from build123d import *

# Parameters (mm, degrees)
F0_W      = 25.4
F0_H      = 50.8
F1_DEPTH  = 50.8
F2_W      = 35.56
F2_H      = 35.56
F3_DEPTH  = 12.7
F4_W      = 17.145
F4_H      = 8.255
F4_H_2    = 6.858
F5_DEPTH  = 7.62
F6_W      = 17.145
F6_H      = 8.255
F6_H_2    = 6.858
F7_DEPTH  = 7.62
F8_W      = 17.145
F8_H      = 35.56
F9_DEPTH  = 7.62
F10_W     = 17.145
F10_H     = 35.56
F11_DEPTH = 7.62


with BuildPart() as f1:
    # F0 (on Front) → F1 (new body)
    with BuildSketch(Plane.XZ):
        with Locations((12.7, 25.4)):
            Rectangle(F0_W, F0_H)
    extrude(amount=F1_DEPTH)

    # F2 (on face) → F3 (cut)
    with BuildSketch(Plane(origin=(0, 0, 0), x_dir=(0, -1, 0), z_dir=(-1, 0, 0))):
        with Locations((25.584483, 25.4)):
            Rectangle(F2_W, F2_H)
    extrude(amount=-F3_DEPTH, mode=Mode.SUBTRACT)

    # F4 (on face) → F5 (cut)
    with BuildSketch(Plane(origin=(0, 0, 0), x_dir=(-1, 0, 0), z_dir=(0, 1, 0))):
        with Locations((-8.5725, 46.6725)):
            Rectangle(F4_W, F4_H)
        with Locations((-8.5725, 32.258)):
            Rectangle(F4_W, F4_H_2)
        with Locations((-8.5725, 18.542)):
            Rectangle(F4_W, F4_H_2)
        with Locations((-8.5725, 4.1275)):
            Rectangle(F4_W, F4_H)
    extrude(amount=-F5_DEPTH, mode=Mode.SUBTRACT)

    # F6 (on face) → F7 (cut)
    with BuildSketch(Plane.XZ.offset(50.8)):
        with Locations((8.5725, 46.6725)):
            Rectangle(F6_W, F6_H)
        with Locations((8.5725, 32.258)):
            Rectangle(F6_W, F6_H_2)
        with Locations((8.5725, 18.542)):
            Rectangle(F6_W, F6_H_2)
        with Locations((8.5725, 4.1275)):
            Rectangle(F6_W, F6_H)
    extrude(amount=-F7_DEPTH, mode=Mode.SUBTRACT)

    # F8 (on face) → F9 (cut)
    with BuildSketch(Plane.XY.offset(50.8)):
        with Locations((8.5725, -25.4)):
            Rectangle(F8_W, F8_H)
    extrude(amount=-F9_DEPTH, mode=Mode.SUBTRACT)

    # F10 (on face) → F11 (cut)
    with BuildSketch(Plane(origin=(0, 0, 0), x_dir=(1, 0, 0), z_dir=(0, 0, -1))):
        with Locations((8.5725, 25.4)):
            Rectangle(F10_W, F10_H)
    extrude(amount=-F11_DEPTH, mode=Mode.SUBTRACT)


solid = f1.part
Build history of the part. All positions in model axes, mm. A direction names the side the tool comes from. Coordinates: 2 decimals unless noted, no trailing zeros. Order: outer loops, then holes, each group sorted by start corner. A loop starts at its lowest first (then second) coordinate and runs counter-clockwise, first axis right, second up. Notation, with made-up numbers: (79, -37) - (100, -37) arc R10 ccw to (100, -30) - close; hole circle Ø9 at (17, -7). An arc over 180 degrees is marked (long way). Write item = value, one per line. Start each with the question number.
1) Wall check: line 1 along Z through (x, y) = (8.75, -4) (3 decimals); line 2 along Y through (x, z) = (12, 26); line 3 along X through (y, z) = (-24.5, 40.5). Give the ranges that are in metal, low to high. Write a range as from..to.
2) Saw through at A-A on x = 5.25. Write the cut outline in (y, z) (3 decimals).
3) Flat gauge pins, fed straight in: pin 1 Ø4 at (y, z) = (-20.5, 8.5) entering from -X; pin 2 Ø2.5 at (x, y) = (6, -4) entering from +Z (3 decimals); pin 3 Ø2.5 at (y, z) = (-17, 48.5) entering from -X (3 decimals). Where does each tip first touch, or does it go through?
4) Saw through at B-B on y = -46. Write the cut outline in (x, z) (3 decimals), then the cut area to 3 significant figures.
5) Saw through at C-C on z = 27. Write the cut outline in (x, y).
6) Two-plate mould, pull along Y, no slides. Class faces 6 (the face through (12.7, -25, 26)), 7 (the face through (15, -43.18, 32)), 8 (the face through (17.145, -47, 32)): pulls with the +Y half, pulls with the -Y half, needs draft (parallel to the pull), parting line crosses it, or undercut.
7) Saw through at D-D on x = 14. Write the cut outline in (y, z) (3 decimals).
8) 3-axis set-ups, long thin cutter, end or side, ignore diameter. For faces 1 (the face through (8, -47, 28.829)), 2 (the face through (6, -43.364, 12)), 3 (the face through (9, -4, 28.829)), 4 (the face through (8, -47, 8.255)), 5 (the face through (14, -25, 7.62)): which of +Z, -Z, +X, -X, +Y, -Y reach the whole face in a straight line?
From the geometry:
q1.line_1 = 8.255..15.113, 21.971..28.829, 35.687..42.545
q1.line_2 = -50.8..-43.36, -7.8..0
q1.line_3 = 12.7..25.4
q2.outline = (-50.8, 8.255) - (-43.364, 8.255) - (-43.364, 15.113) - (-50.8, 15.113) - close; (-50.8, 21.971) - (-43.364, 21.971) - (-43.364, 28.829) - (-50.8, 28.829) - close; (-50.8, 35.687) - (-43.364, 35.687) - (-43.364, 42.545) - (-50.8, 42.545) - close; (-7.804, 7.62) - (-7.62, 7.62) - (-7.62, 8.255) - (0, 8.255) - (0, 15.113) - (-7.62, 15.113) - (-7.62, 21.971) - (0, 21.971) - (0, 28.829) - (-7.62, 28.829) - (-7.62, 35.687) - (0, 35.687) - (0, 42.545) - (-7.62, 42.545) - (-7.62, 43.18) - (-7.804, 43.18) - close
q3.pin_1 = 12.7
q3.pin_2 = 42.545
q3.pin_3 = 17.145
q4.outline = (0, 8.255) - (17.145, 8.255) - (17.145, 0) - (25.4, 0) - (25.4, 50.8) - (17.145, 50.8) - (17.145, 42.545) - (0, 42.545) - (0, 35.687) - (17.145, 35.687) - (17.145, 28.829) - (0, 28.829) - (0, 21.971) - (17.145, 21.971) - (17.145, 15.113) - (0, 15.113) - close
q4.area = 772 mm^2
q5.outline = (0, -50.8) - (25.4, -50.8) - (25.4, 0) - (0, 0) - (0, -7.8) - (12.7, -7.8) - (12.7, -43.36) - (0, -43.36) - close
q6.face_6 = undercut
q6.face_7 = pulls with the -Y half
q6.face_8 = needs draft
q7.outline = (-50.8, 8.255) - (-43.18, 8.255) - (-43.18, 7.62) - (-7.62, 7.62) - (-7.62, 8.255) - (0, 8.255) - (0, 15.113) - (-7.62, 15.113) - (-7.62, 21.971) - (0, 21.971) - (0, 28.829) - (-7.62, 28.829) - (-7.62, 35.687) - (0, 35.687) - (0, 42.545) - (-7.62, 42.545) - (-7.62, 43.18) - (-43.18, 43.18) - (-43.18, 42.545) - (-50.8, 42.545) - (-50.8, 35.687) - (-43.18, 35.687) - (-43.18, 28.829) - (-50.8, 28.829) - (-50.8, 21.971) - (-43.18, 21.971) - (-43.18, 15.113) - (-50.8, 15.113) - close
q8.face_1 = -X, -Y
q8.face_2 = +Z, -Z, -X
q8.face_3 = -X, +Y
q8.face_4 = -Z, -X, -Y
q8.face_5 = -Z, -X, +Y, -Y
